```python
from build123d import *

# Parameters (mm, degrees)
FILLET_1_R = 0.5
FILLET_2_R = 0.2


with BuildPart() as part:
    # 草图1 → 旋转4 (revolve)
    with BuildSketch(Plane.XY, mode=Mode.PRIVATE) as revolve_4_sk:
        with BuildLine():
            Line((4.043760626, 8), (7.5, 8))
            Line((7.5, 8), (7.5, 7))
            Line((7.5, 7), (6.5, 7))
            Line((6.5, 7), (6.5, 0))
            Line((6.5, 0), (0, 0))
            Line((0, 0), (0, 10.8))
            ThreePointArc((0, 10.8), (2.459268184, 10.031675661), (4.043760626, 8))
        make_face()
    revolve(revolve_4_sk.sketch.rotate(Axis((0, 28.404003486, 0), (0, -1, 0)), 180), axis=Axis((0, 28.404003486, 0), (0, -1, 0)))

    # 圆角1
    fillet_1_edges = [part.edges().sort_by_distance(p)[0] for p in [
        (6.5, 0, 0),
    ]]
    fillet(fillet_1_edges, radius=FILLET_1_R)

    # 圆角2
    fillet_2_edges = [part.edges().sort_by_distance(p)[0] for p in [
        (7.5, 8, 0),
        (7.5, 7, 0),
    ]]
    fillet(fillet_2_edges, radius=FILLET_2_R)


solid = part.part
```
Geometry: final body of the model. Coordinates: model frame, mm. A direction names the side the tool comes from. Round coordinates to 2 decimals unless told otherwise and drop trailing zeros. Write each loop counter-clockwise with the first axis right and the second up, starting at its lowest first coordinate (ties: lowest second). Pieces come first, ordered by that corner, then holes. Notation, with made-up numbers: M 69.25,70 L 107.25,70 A33 cw 107.25,105 Z; hole C -36,21.5 d3. An arc over 180 degrees is marked long. Answer in a Markdown table with one row per item. Add a question column.
(1) Reachability of faces 1 (the face through (7, 7, 1)), 2 (the face through (3, 8, 3)), 3 (the face through (-4.032, 7.496, -6.324)) from +Z, -Z, +X, -X, +Y, -Y: full face, straight path, thin tool, end or side. Return the list, or none.
(2) Cut plane A-A, the plane x = 0. Return the cut outline in (y, z).
(3) Contact query for flat-ended pins moving along their axis: pin 1 (3 mm diameter, centred on x = 5.5, y = 2, fed in from -Z); pin 2 (6 mm diameter, centred on x = -2, y = 2.5, fed in from +Z); pin 3 (4 mm diameter, centred on x = 5, z = -5, fed in from +Y); pin 4 (1.5 mm diameter, centred on x = 6, y = 9, fed in from -Z) (1 decimal). Output: stop coordinate, or through.
(4) Cut plane D-D, the plane y = 8.25. Return the cut outline in (x, z), then the cut area to 3 significant figures.
(5) Cut plane C-C, the plane y = 6.5. Return the cut outline in (x, z), then the cut area to 3 significant figures.
(6) Cut plane B-B, the plane z = 0. Return the cut outline in (x, y).
(7) Ray query, L1, parallel to Y at x = -3.25, z = -4.25; L2, parallel to X at y = 2, z = 0.25; L3, parallel to Y at x = 2.75, z = -6. Return the intervals inside material, ascending.
Established:
| question | item | result |
|---|---|---|
| 1 | face 1 | -Y |
| 1 | face 2 | +Y |
| 1 | face 3 | +Y, -Y |
| 2 | outline | M 0,-6 A0.5 ccw 0.5,-6.5 L 7,-6.5 L 7,-7.3 A0.2 ccw 7.2,-7.5 L 7.8,-7.5 A0.2 ccw 8,-7.3 L 8,-4.04 A4.32 ccw 8,4.04 L 8,7.3 A0.2 ccw 7.8,7.5 L 7.2,7.5 A0.2 ccw 7,7.3 L 7,6.5 L 0.5,6.5 A0.5 ccw 0,6 Z |
| 3 | pin 1 | z = -5.12 |
| 3 | pin 2 | z = 6.5 |
| 3 | pin 3 | y = 8 |
| 3 | pin 4 | through |
| 4 | outline | C 0,0 d7.88 |
| 4 | area | 48.8 mm² |
| 5 | outline | C 0,0 d13 |
| 5 | area | 133 mm² |
| 6 | outline | M -7.5,7.2 A0.2 ccw -7.3,7 L -6.5,7 L -6.5,0.5 A0.5 ccw -6,0 L 6,0 A0.5 ccw 6.5,0.5 L 6.5,7 L 7.3,7 A0.2 ccw 7.5,7.2 L 7.5,7.8 A0.2 ccw 7.3,8 L 4.04,8 A4.32 ccw -4.04,8 L -7.3,8 A0.2 ccw -7.5,7.8 Z |
| 7 | L1 | 0 to 8 |
| 7 | L2 | -6.5 to 6.5 |
| 7 | L3 | 7 to 8 |
